Check sheet for the drawn part. Datum: minimum x, y, z corner. Units: mm. A direction names the side the tool comes from. Coordinates: 2 decimals unless noted, no trailing zeros. Order: outer loops, then holes, each group sorted by start corner. A loop starts at its lowest first (then second) coordinate and runs counter-clockwise, first axis right, second up.
1. Cross-section at B-B (x = 5.25). Enter the section's corners in (y, z).
2. Draft check along X on the marked faces 3, 4 and 5. Enter one of: released by +X, released by -X, zero draft, split by the parting line, or undercut.
3. Cross-section at A-A (z = 2.5). Enter the section's corners in (x, y), then the cut area to 3 significant figures.
4. Set-up check for the marked faces 1 and 2: record each of +Z, -Z, +X, -X, +Y, -Y from which the full face is reachable in a straight line by a thin tool's end or side.
5. Cross-section at C-C (y = 92). Enter the section's corners in (x, z).
6. Cross-section at D-D (y = 32). Enter the section's corners in (x, z).
7. Thickness scan on line 1 (Y direction, x = 5.25, z = 0.75); line 2 (X direction, y = 6.5, z = 1.5); line 3 (Y direction, x = 6, z = 0.75). Record the ranges inside material, lowest first.
8. Gauge pin test, flat end, axial feed: pin 1 Ø2.5 at (x, y) = (6.5, 32) entering from +Z. Record the tip position at first contact, or that the pin passes through.
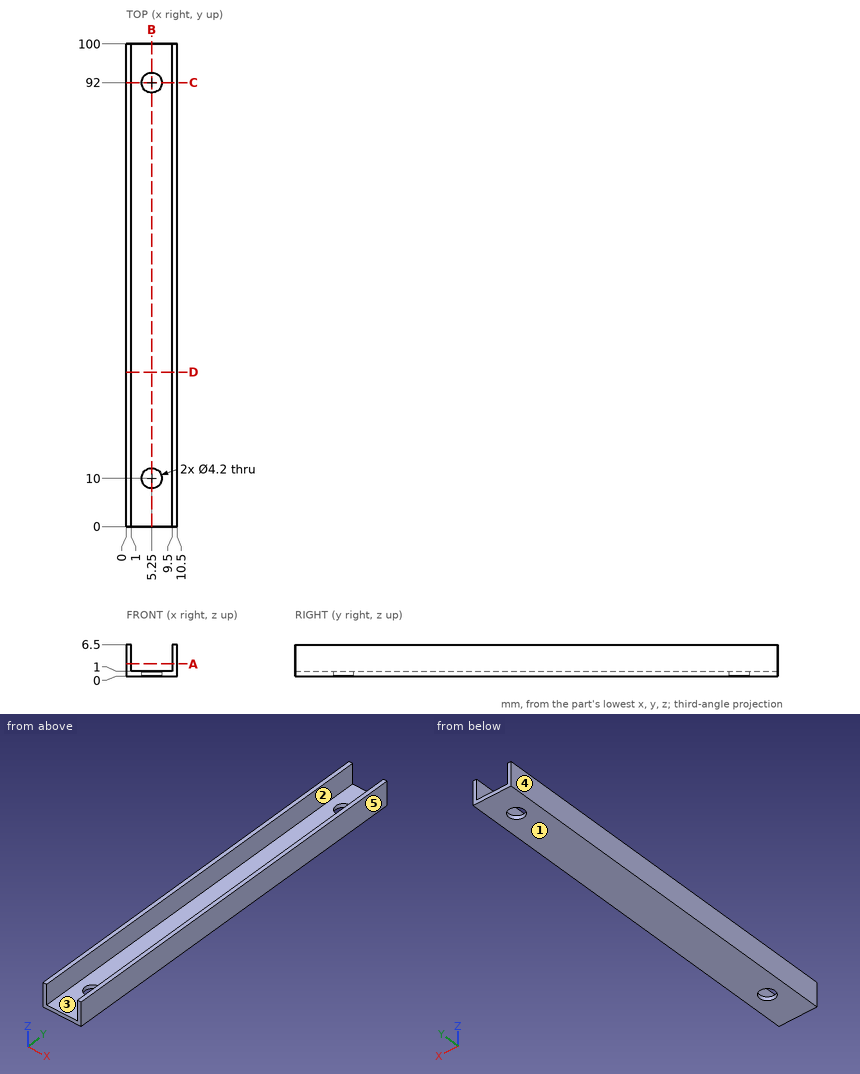
Data:
1. outline: (0, 0) - (7.9, 0) - (7.9, 1) - (0, 1) - close; (12.1, 0) - (89.9, 0) - (89.9, 1) - (12.1, 1) - close; (94.1, 0) - (100, 0) - (100, 1) - (94.1, 1) - close
2. face 3: undercut
2. face 4: released by -X
2. face 5: released by +X
3. outline: (0, 0) - (1, 0) - (1, 100) - (0, 100) - close; (9.5, 0) - (10.5, 0) - (10.5, 100) - (9.5, 100) - close
3. area: 200 mm2
4. face 1: -Z, +X, -X, +Y, -Y
4. face 2: +Z, +Y, -Y
5. outline: (0, 0) - (3.15, 0) - (3.15, 1) - (1, 1) - (1, 6.5) - (0, 6.5) - close; (7.35, 0) - (10.5, 0) - (10.5, 6.5) - (9.5, 6.5) - (9.5, 1) - (7.35, 1) - close
6. outline: (0, 0) - (10.5, 0) - (10.5, 6.5) - (9.5, 6.5) - (9.5, 1) - (1, 1) - (1, 6.5) - (0, 6.5) - close
7. line 1: y = 0 to 7.9, 12.1 to 89.9, 94.1 to 100
7. line 2: x = 0 to 1, 9.5 to 10.5
7. line 3: y = 0 to 8.04, 11.96 to 90.04, 93.96 to 100
8. pin 1: stops at z = 1
